from build123d import *

# Parameters (mm, degrees)
SALIENTE_EXTRUIR1_DEPTH = 23
SALIENTE_EXTRUIR2_DEPTH = 2
CROQUIS3_W              = 74.8935
CROQUIS3_H              = 50
SALIENTE_EXTRUIR3_DEPTH = 2
CROQUIS4_R              = 4.05
SALIENTE_EXTRUIR4_DEPTH = 50
CHAFL_N2_SIZE           = 1
CROQUIS7_R              = 4.05
CROQUIS7_R_2            = 13.05
SALIENTE_EXTRUIR5_DEPTH = 6
CROQUIS8_W              = 12
CROQUIS8_H              = 4
SALIENTE_EXTRUIR6_DEPTH = 16
REDONDEO3_R             = 2
REDONDEO4_R             = 5
CROQUIS14_R             = 4
CORTAR_EXTRUIR1_DEPTH   = 10
SALIENTE_EXTRUIR7_DEPTH = 1
CROQUIS20_R             = 4.05
CROQUIS20_R_2           = 10
SALIENTE_EXTRUIR8_DEPTH = 2
CHAFL_N3_SIZE           = 1
CROQUIS22_R             = 5.05
CROQUIS22_R_2           = 15
CORTAR_EXTRUIR3_DEPTH   = 5
REDONDEO6_R             = 1


with BuildPart() as part:
    # Croquis1 → Saliente-Extruir1 (new, symmetric)
    with BuildSketch(Plane.XY):
        Polygon((-7.48935, 0), (7.48935, 0), (0.00065, 21.6199), align=None)
    extrude(amount=SALIENTE_EXTRUIR1_DEPTH, both=True)

    # Croquis2 → Saliente-Extruir2 (add)
    with BuildSketch(Plane.XY.offset(23)):
        Polygon((37.44675, 0), (-37.44675, 0), (0.00065, 21.6199), align=None)
    saliente_extruir2 = extrude(amount=SALIENTE_EXTRUIR2_DEPTH)

    # Simetría1: Saliente-Extruir2 across plane
    add(saliente_extruir2.mirror(Plane.XY))

    # Croquis3 → Saliente-Extruir3 (add)
    with BuildSketch(Plane.XZ):
        Rectangle(CROQUIS3_W, CROQUIS3_H)
    extrude(amount=SALIENTE_EXTRUIR3_DEPTH)

    # Croquis4 → Saliente-Extruir4 (add)
    with BuildSketch(Plane.XY.offset(25)):
        with BuildLine():
            Line((7.743545699, -2), (-7.743545699, -2))
            ThreePointArc((-7.743545699, -2), (-6.147743753, -2.794422898), (-5.819683414, -4.546583851))
            ThreePointArc((-5.819683414, -4.546583851), (0, -12.25), (5.819683414, -4.546583851))
            ThreePointArc((5.819683414, -4.546583851), (6.147743753, -2.794422898), (7.743545699, -2))
        make_face()
        with Locations((0, -6.2)):
            Circle(CROQUIS4_R, mode=Mode.SUBTRACT)
    extrude(amount=-SALIENTE_EXTRUIR4_DEPTH)

    # Chaflán2
    chafl_n2_edges = [part.edges().sort_by_distance(p)[0] for p in [
        (-4.05, -6.2, -25),
        (-4.05, -6.2, 25),
    ]]
    chamfer(chafl_n2_edges, length=CHAFL_N2_SIZE)


with BuildPart() as body_2:
    # Croquis7 → Saliente-Extruir5 (new body)
    with BuildSketch(Plane(origin=(0, 0, -25), x_dir=(-1, 0, 0), z_dir=(0, 0, -1))):
        with BuildLine():
            Line((-9.986152883, 8.775872282), (-42.60542858, -12.975186214))
            ThreePointArc((-42.60542858, -12.975186214), (-44.239992249, -14.776089142), (-44.831497223, -17.135150737))
            Line((-44.831497223, -17.135150737), (-44.831497223, -35.665252187))
            Line((-44.831497223, -35.665252187), (44.831497223, -35.665252187))
            Line((44.831497223, -35.665252187), (44.831497223, -17.135150737))
            ThreePointArc((44.831497223, -17.135150737), (44.239992249, -14.776089142), (42.60542858, -12.975186214))
            Line((42.60542858, -12.975186214), (9.986152883, 8.775872282))
            ThreePointArc((9.986152883, 8.775872282), (0, 11.8), (-9.986152883, 8.775872282))
        make_face()
        with Locations((-27, -21.615252187)):
            Circle(CROQUIS7_R, mode=Mode.SUBTRACT)
        with Locations(Location((27, -21.615252187, 0), (0, 0, 180))):
            Circle(CROQUIS7_R, mode=Mode.SUBTRACT)
        with Locations((0, -6.2)):
            Circle(CROQUIS7_R_2, mode=Mode.SUBTRACT)
    extrude(amount=SALIENTE_EXTRUIR5_DEPTH)

    # Croquis8 → Saliente-Extruir6 (add)
    with BuildSketch(Plane.XY.offset(-25)):
        with Locations((-16, -33.665252187)):
            Rectangle(CROQUIS8_W, CROQUIS8_H)
        with Locations((16, -33.665252187)):
            Rectangle(CROQUIS8_W, CROQUIS8_H)
    extrude(amount=SALIENTE_EXTRUIR6_DEPTH)

    # Redondeo3
    redondeo3_edges = [body_2.edges().sort_by_distance(p)[0] for p in [
        (-22, -33.665252187, -25),
        (-10, -33.665252187, -25),
        (22, -33.665252187, -25),
        (10, -33.665252187, -25),
    ]]
    fillet(redondeo3_edges, radius=REDONDEO3_R)

    # Redondeo4
    redondeo4_edges = [body_2.edges().sort_by_distance(p)[0] for p in [
        (-22, -33.665252187, -9),
        (-10, -33.665252187, -9),
        (22, -33.665252187, -9),
        (10, -33.665252187, -9),
    ]]
    fillet(redondeo4_edges, radius=REDONDEO4_R)

    # Croquis14 → Cortar-Extruir1 (cut)
    with BuildSketch(Plane(origin=(0, -31.665252187, 0), x_dir=(1, 0, 0), z_dir=(0, 1, 0))):
        with Locations(Location((-16, 15, 0), (0, 0, 270))):
            Circle(CROQUIS14_R)
        with Locations(Location((16, 15, 0), (0, 0, 270))):
            Circle(CROQUIS14_R)
    extrude(amount=-CORTAR_EXTRUIR1_DEPTH, mode=Mode.SUBTRACT)

    # Croquis3D2 → Saliente-Extruir7 (add, symmetric, along a direction that is not the sketch's normal)
    with BuildSketch(Plane(origin=(-16, -31.665252187, -22.681195735), x_dir=(0.03434705256799914, 0.973825325774171, -0.22468759391813525), z_dir=(-0.9993785848148502, 0.035248322136908906, 0))):
        Polygon((0, 0), (10.320125934, 0), (0.521006551, 2.259514415), align=None)
    saliente_extruir7 = extrude(amount=SALIENTE_EXTRUIR7_DEPTH, dir=(-1, 0, 0), both=True)

    # Simetría2: Saliente-Extruir7 across plane
    add(saliente_extruir7.mirror(Plane(origin=(0, 0, 0), x_dir=(0, 0, 1), z_dir=(1, 0, 0))))

    # Croquis20 → Saliente-Extruir8 (add)
    with BuildSketch(Plane(origin=(0, 0, -31), x_dir=(-1, 0, 0), z_dir=(0, 0, -1))):
        with BuildLine():
            Line((42.60542858, -12.975186214), (9.986152883, 8.775872282))
            ThreePointArc((9.986152883, 8.775872282), (0, 11.8), (-9.986152883, 8.775872282))
            Line((-9.986152883, 8.775872282), (-42.60542858, -12.975186214))
            ThreePointArc((-42.60542858, -12.975186214), (-44.239992249, -14.776089142), (-44.831497223, -17.135150737))
            Line((-44.831497223, -17.135150737), (-44.831497223, -35.665252187))
            Line((-44.831497223, -35.665252187), (44.831497223, -35.665252187))
            Line((44.831497223, -35.665252187), (44.831497223, -17.135150737))
            ThreePointArc((44.831497223, -17.135150737), (44.239992249, -14.776089142), (42.60542858, -12.975186214))
        make_face()
        with Locations((-27, -21.615252187)):
            Circle(CROQUIS20_R, mode=Mode.SUBTRACT)
        with Locations(Location((27, -21.615252187, 0), (0, 0, 180))):
            Circle(CROQUIS20_R, mode=Mode.SUBTRACT)
        with Locations((0, -6.2)):
            Circle(CROQUIS20_R_2, mode=Mode.SUBTRACT)
    extrude(amount=SALIENTE_EXTRUIR8_DEPTH)

    # Chaflán3
    chafl_n3_edges = [body_2.edges().sort_by_distance(p)[0] for p in [
        (31.05, -21.615252187, -33),
        (-31.05, -21.615252187, -33),
    ]]
    chamfer(chafl_n3_edges, length=CHAFL_N3_SIZE)

    # Croquis22 → Cortar-Extruir3 (cut)
    # profile 1 of 3: a face of its own
    with BuildSketch(Plane(origin=(0, 0, -33), x_dir=(-1, 0, 0), z_dir=(0, 0, -1))):
        with BuildLine():
            ThreePointArc((44.831497223, -17.135150737), (44.239992249, -14.776089142), (42.60542858, -12.975186214))
            Line((42.60542858, -12.975186214), (9.986152883, 8.775872282))
            ThreePointArc((9.986152883, 8.775872282), (0, 11.8), (-9.986152883, 8.775872282))
            Line((-9.986152883, 8.775872282), (-42.60542858, -12.975186214))
            ThreePointArc((-42.60542858, -12.975186214), (-44.239992249, -14.776089142), (-44.831497223, -17.135150737))
            Line((-44.831497223, -17.135150737), (-44.831497223, -35.665252187))
            Line((-44.831497223, -35.665252187), (44.831497223, -35.665252187))
            Line((44.831497223, -35.665252187), (44.831497223, -17.135150737))
        make_face()
        with Locations((-27, -21.615252187)):
            Circle(CROQUIS22_R, mode=Mode.SUBTRACT)
        with Locations((27, -21.615252187)):
            Circle(CROQUIS22_R, mode=Mode.SUBTRACT)
        with Locations((0, -6.2)):
            Circle(CROQUIS22_R_2, mode=Mode.SUBTRACT)
    # profile 2 of 3: a face of its own
    with BuildSketch(Plane(origin=(0, 0, -33), x_dir=(-1, 0, 0), z_dir=(0, 0, -1))):
        with Locations((-27, -21.615252187)):
            Circle(CROQUIS22_R)
    # profile 3 of 3: a face of its own
    with BuildSketch(Plane(origin=(0, 0, -33), x_dir=(-1, 0, 0), z_dir=(0, 0, -1))):
        with Locations((27, -21.615252187)):
            Circle(CROQUIS22_R)
    extrude(amount=-CORTAR_EXTRUIR3_DEPTH, mode=Mode.SUBTRACT)

    # Redondeo6
    redondeo6_edges = [body_2.edges().sort_by_distance(p)[0] for p in [
        (15, -6.2, -33),
        (15, -6.2, -28),
    ]]
    fillet(redondeo6_edges, radius=REDONDEO6_R)


solid = body_2.part
Check sheet for the modelled part. Datum: model origin and axes. Units: mm. A direction names the side the tool comes from. Give positions to 0.01 mm unless a question says otherwise; leave off trailing zeros. Loops run counter-clockwise (first coordinate to the right, second up) from the corner with the lowest first, then second, coordinate; pieces in that order, holes last. Notation, with made-up numbers: M 11,-33 L 66,-33 A24 ccw 66,-20 Z; hole C -5,-4 d10. An arc over 180 degrees is marked long. Return JSON: item names as keys, results as strings. Group by question number.
1. Cross-section at C-C on z = -15. Record the boundary of the cut face in (x, y).
2. Cross-section at D-D on y = -28. Record the boundary of the cut face in (x, z), plus the area to 3 significant figures.
3. Go/stop test with flat-tipped pins: pin 1 (7 mm diameter, centred on x = 16, z = -15, fed in from +Y); pin 2 (9.5 mm diameter, centred on x = 27, y = -21.62, fed in from +Z); pin 3 (2 mm diameter, centred on y = -34.5, z = -17, fed in from -X); pin 4 (3 mm diameter, centred on y = -33, z = -18.5, fed in from +X). Record where each tip stops, or that it passes through.
4. Mould release check, pull along Y, two halves, no side actions. Record for faces 1 (the cylindrical face through (-0.1, 11.8, -26.5)), 2 (the flat face through (22, -34, -19)), 3 (the cylindrical face through (15, -6, -31)), 4 (the cylindrical face through (23.137, -20.399, -26.479)): released by +Y, released by -Y, zero draft, split by the parting line, or undercut.
5. Thickness scan on L1, parallel to X at y = -34, z = -15; L2, parallel to Z at x = 15, y = 4; L3, parallel to Y at x = -16, z = -19.5. Record the ranges inside material, lowest first.
6. Cross-section at A-A on z = -20.5. Record the boundary of the cut face in (x, y).
7. Cross-section at B-B on x = 0. Record the boundary of the cut face in (y, z).
8. Tool access check on faces 5 (the cylindrical face through (9.4, -33.64, -24.43)), 6 (the flat face through (3, -16, -31)), 7 (the flat face through (-22, -34, -19)), 8 (the flat face through (-15.839, -26.711, -23.824)). Record the directions out of +Z, -Z, +X, -X, +Y, -Y that give a thin tool (end or side, any length) a straight path to the whole face; none if there is none.
Return value:
{
 "1": {"outline": "M -22,-35.67 L -20,-35.67 L -20,-31.67 L -22,-31.67 Z; M -12,-35.67 L -10,-35.67 L -10,-31.67 L -12,-31.67 Z; M 10,-35.67 L 12,-35.67 L 12,-31.67 L 10,-31.67 Z; M 20,-35.67 L 22,-35.67 L 22,-31.67 L 20,-31.67 Z"},
 "2": {"outline": "M -44.83,-28 L 44.83,-28 L 44.83,-25 L 16.87,-25 L 16.87,-23.53 L 14.87,-23.53 L 14.87,-25 L -14.87,-25 L -14.87,-23.53 L -16.87,-23.53 L -16.87,-25 L -44.83,-25 Z", "area": "275 mm^2"},
 "3": {"pin 1": "through", "pin 2": "z = -25", "pin 3": "x = -22", "pin 4": "x = 22"},
 "4": {"face 1": "released by +Y", "face 2": "zero draft", "face 3": "split by the parting line", "face 4": "undercut"},
 "5": {"L1": "-22 to -20, -12 to -10, 10 to 12, 20 to 22", "L2": "-28 to -25", "L3": "-35.67 to -31.67"},
 "6": {"outline": "M -22,-35.67 L -10,-35.67 L -10,-31.67 L -22,-31.67 Z; M 10,-35.67 L 22,-35.67 L 22,-31.67 L 10,-31.67 Z"},
 "7": {"outline": "M -35.67,-28 L -22.2,-28 A1 cw -21.2,-29 L -21.2,-32 A1 ccw -20.2,-33 L -16.2,-33 L -16.2,-31 L -19.25,-31 L -19.25,-25 L -35.67,-25 Z; M 3.8,-33 L 7.8,-33 A1 ccw 8.8,-32 L 8.8,-29 A1 cw 9.8,-28 L 11.8,-28 L 11.8,-25 L 6.85,-25 L 6.85,-31 L 3.8,-31 Z"},
 "8": {"face 5": "+Z, +Y, -Y", "face 6": "+Z", "face 7": "+Z, -X, +Y, -Y", "face 8": "+Z, +X, -X, +Y"}
}
